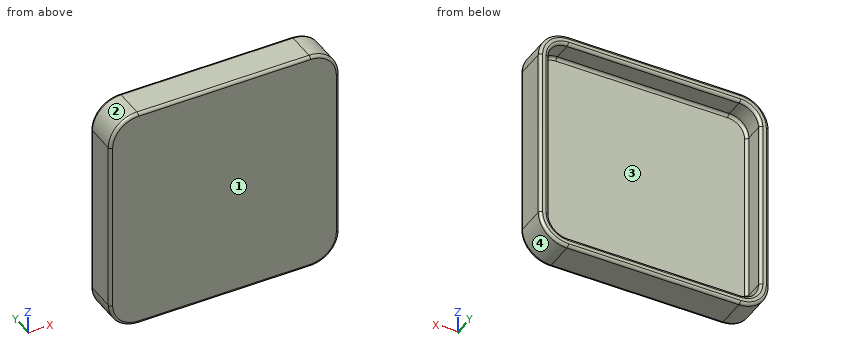
from build123d import *

# Parameters (mm, degrees)
BOSS_EXTRUDE1_DEPTH = 2
EXTRUDE_THIN1_START = 2
EXTRUDE_THIN1_DEPTH = 4
FILLET1_R           = 0.5


with BuildPart() as part:
    # Sketch1 → Boss-Extrude1 (new body)
    with BuildSketch(Plane(origin=(0, 0, 0), x_dir=(1, 0, 0), z_dir=(0, 1, 0))):
        with BuildLine():
            Line((-15, 20), (15, 20))
            ThreePointArc((15, 20), (18.535533906, 18.535533906), (20, 15))
            Line((20, 15), (20, -15))
            ThreePointArc((20, -15), (18.535533906, -18.535533906), (15, -20))
            Line((15, -20), (-15, -20))
            ThreePointArc((-15, -20), (-18.535533906, -18.535533906), (-20, -15))
            Line((-20, -15), (-20, 15))
            ThreePointArc((-20, 15), (-18.535533906, 18.535533906), (-15, 20))
        make_face()
    extrude(amount=BOSS_EXTRUDE1_DEPTH)

    # Sketch1<2> → Extrude-Thin1 (add)
    with BuildSketch(Plane(origin=(0, 0, 0), x_dir=(1, 0, 0), z_dir=(0, 1, 0)).offset(EXTRUDE_THIN1_START)):
        with BuildLine():
            Line((15, -20), (-15, -20))
            ThreePointArc((-15, -20), (-18.535533906, -18.535533906), (-20, -15))
            Line((-20, -15), (-20, 15))
            ThreePointArc((-20, 15), (-18.535533906, 18.535533906), (-15, 20))
            Line((-15, 20), (15, 20))
            ThreePointArc((15, 20), (18.535533906, 18.535533906), (20, 15))
            Line((20, 15), (20, -15))
            ThreePointArc((20, -15), (18.535533906, -18.535533906), (15, -20))
        make_face()
        with BuildLine():
            Line((15, -18.4), (-15, -18.4))
            ThreePointArc((-15, -18.4), (-17.404163056, -17.404163056), (-18.4, -15))
            Line((-18.4, -15), (-18.4, 15))
            ThreePointArc((-18.4, 15), (-17.404163056, 17.404163056), (-15, 18.4))
            Line((-15, 18.4), (15, 18.4))
            ThreePointArc((15, 18.4), (17.404163056, 17.404163056), (18.4, 15))
            Line((18.4, 15), (18.4, -15))
            ThreePointArc((18.4, -15), (17.404163056, -17.404163056), (15, -18.4))
        make_face(mode=Mode.SUBTRACT)
    extrude(amount=EXTRUDE_THIN1_DEPTH)

    # Fillet1
    fillet1_edges = [part.edges().sort_by_distance(p)[0] for p in [
        (0, 0, 20),
        (-18.535533906, 0, 18.535533906),
        (-18.535533906, 6, -18.535533906),
        (-18.535533906, 6, 18.535533906),
        (18.535533906, 6, 18.535533906),
        (18.535533906, 6, -18.535533906),
        (-18.4, 6, 0),
        (0, 6, -18.4),
        (18.4, 6, 0),
        (0, 6, 18.4),
        (-17.404163056, 2, -17.404163056),
        (-17.404163056, 2, 17.404163056),
        (17.404163056, 2, 17.404163056),
        (17.404163056, 2, -17.404163056),
        (-20, 6, 0),
        (0, 6, 20),
        (20, 6, 0),
        (0, 6, -20),
        (-17.404163056, 6, -17.404163056),
        (-18.4, 2, 0),
        (-17.404163056, 6, 17.404163056),
        (0, 2, 18.4),
        (17.404163056, 6, 17.404163056),
        (18.4, 2, 0),
        (17.404163056, 6, -17.404163056),
        (0, 2, -18.4),
        (-20, 0, 0),
        (-18.535533906, 0, -18.535533906),
        (0, 0, -20),
        (18.535533906, 0, -18.535533906),
        (20, 0, 0),
        (18.535533906, 0, 18.535533906),
    ]]
    fillet(fillet1_edges, radius=FILLET1_R)


solid = part.part
Can you work these out from the model? Positions are in its coordinate system, mm. Face numbers are marked on the shaded views. Round coordinates to 2 decimals unless told otherwise and drop trailing zeros. Loops run counter-clockwise (first coordinate to the right, second up) from the corner with the lowest first, then second, coordinate; pieces in that order, holes last. Notation, with made-up numbers: (-40, 57) - (17, 57) arc R25 cw to (17, 90) - close; hole circle Ø7 at (49, 27). An arc over 180 degrees is marked (long way). Use CSV: the item, a comma, the result in double quotes. Start each with the question number.
1) Please list where these lines run through material, in increasing order: probe 1 along X at (y, z) = (2.55, -1.5); probe 2 along Y at (x, z) = (-16.5, 2). Write a range as [from, to].
2) If we section it at C-C on z = -8: Write out the boundary of the cut face in (x, y), plus the area to 3 significant figures.
3) For pin 1 Ø10.5 at (x, z) = (-8.5, 4) entering from +Y, with a flat end and sliding along its axis, tell me the tip position at first contact or that it passes through.
4) If we section it at B-B on x = -10: Write out the boundary of the cut face in (y, z).
5) We'd pull the mould along X, two halves only. Please class the marked faces 1, 2, 3 and 4: released by +X, released by -X, zero draft, split by the parting line, or undercut.
6) If we section it at A-A on y = 3.4: Write out the boundary of the cut face in (x, z), plus the area to 3 significant figures.
Geometry results:
1,probe 1,"x = [-20, -18.4], [18.4, 20]"
1,probe 2,"y = [0, 2]"
2,outline,"(-20, 0.5) arc R0.5 ccw to (-19.5, 0) - (19.5, 0) arc R0.5 ccw to (20, 0.5) - (20, 5.5) arc R0.5 ccw to (19.5, 6) - (18.9, 6) arc R0.5 ccw to (18.4, 5.5) - (18.4, 2.5) arc R0.5 cw to (17.9, 2) - (-17.9, 2) arc R0.5 cw to (-18.4, 2.5) - (-18.4, 5.5) arc R0.5 ccw to (-18.9, 6) - (-19.5, 6) arc R0.5 ccw to (-20, 5.5) - close"
2,area,"92.6 mm2"
3,pin 1,"stops at y = 2"
4,outline,"(0, -19.5) arc R0.5 ccw to (0.5, -20) - (5.5, -20) arc R0.5 ccw to (6, -19.5) - (6, -18.9) arc R0.5 ccw to (5.5, -18.4) - (2.5, -18.4) arc R0.5 cw to (2, -17.9) - (2, 17.9) arc R0.5 cw to (2.5, 18.4) - (5.5, 18.4) arc R0.5 ccw to (6, 18.9) - (6, 19.5) arc R0.5 ccw to (5.5, 20) - (0.5, 20) arc R0.5 ccw to (0, 19.5) - close"
5,face 1,"zero draft"
5,face 2,"released by -X"
5,face 3,"undercut"
5,face 4,"released by +X"
6,outline,"(-20, -15) arc R5 ccw to (-15, -20) - (15, -20) arc R5 ccw to (20, -15) - (20, 15) arc R5 ccw to (15, 20) - (-15, 20) arc R5 ccw to (-20, 15) - close; hole (-18.4, -15) arc R3.4 ccw to (-15, -18.4) - (15, -18.4) arc R3.4 ccw to (18.4, -15) - (18.4, 15) arc R3.4 ccw to (15, 18.4) - (-15, 18.4) arc R3.4 ccw to (-18.4, 15) - close"
6,area,"234 mm2"
